Source: CAD feature listing. Evaluate the final solid. Frame: model axes, mm. A direction names the side the tool comes from. Round coordinates to 2 decimals unless told otherwise and drop trailing zeros. Loops run counter-clockwise (first coordinate to the right, second up) from the corner with the lowest first, then second, coordinate; pieces in that order, holes last. Notation, with made-up numbers: M 1,-28.75 L 32,-28.75 A18 cw 32,-19.75 Z; hole C 7,-37 d9. An arc over 180 degrees is marked long. Write each question's results on one line, items separated by ' | '. Start each with the question number.
1. Section B-B on x = 0. Output: boundary loops of the cut face in (y, z), and give its area (3 significant figures).
2. Set-up query: faces 1 (the flat face through (-1, 1, 3)), 2 (the flat face through (12.5, -5, -1)), 3 (the flat face through (-12.5, -5, -1)), 4 (the flat face through (12.5, 13, 1)). Return all of +Z, -Z, +X, -X, +Y, -Y with unobstructed straight access to the full face (end or side cutting, diameter ignored); none if empty.
3. Contact query for flat-ended pins moving along their axis: pin 1 Ø24 at (x, y) = (16, -10) entering from -Z; pin 2 Ø1 at (y, z) = (19, 1.5) entering from -X; pin 3 Ø2 at (y, z) = (29.5, 0.5) entering from -X; pin 4 Ø2.5 at (x, z) = (5.5, 1) entering from +Y. Output: stop coordinate, or through.
4. Section D-D on y = 12.5. Output: boundary loops of the cut face in (x, z), and give its area (3 significant figures).
5. Draft query along Y for faces 5 (the flat face through (0, 4, -1)), 6 (the flat face through (0, -5, -2)), 7 (the flat face through (0, 16.5, 1)), 8 (the flat face through (0, -14.5, -1)). Return one class per face: released by +Y, released by -Y, zero draft, split by the parting line, or undercut.
6. Section A-A on y = 0. Output: boundary loops of the cut face in (x, z).
7. Ray query, line 1 (X direction, y = 0, z = -0.45); line 2 (Y direction, x = -10.5, z = -0.2); line 3 (X direction, y = -12.5, z = 1.4). Return the intervals inside material, ascending.
8. Section C-C on z = -0.9. Output: boundary loops of the cut face in (x, y).
from build123d import *

# Parameters (mm, degrees)
ESQUISSE1_R                  = 40
ESQUISSE1_R_2                = 1.05
BOSS_EXTRU_1_DEPTH           = 3
ESQUISSE2_W                  = 25
ESQUISSE2_H                  = 7
ENL_V_MAT_EXTRU_4_DEPTH      = 14
BOSS_EXTRU_6_DEPTH           = 2
ENL_V_MAT_EXTRU_5_DEPTH      = 2
ESQUISSE2_9_W                = 12.5
ESQUISSE2_9_H                = 18.5
BOSS_EXTRU_7_DEPTH           = 2
ENL_V_MAT_EXTRU_6_DEPTH      = 57.648036153
ENL_V_MAT_EXTRU_6_DEPTH_BACK = 57.648036153
ESQUISSE7_R                  = 1.05


with BuildPart() as part:
    # Esquisse1 → Boss.-Extru.1 (new body)
    with BuildSketch(Plane.XY):
        Circle(ESQUISSE1_R)
        with Locations((-10.5, -12.5)):
            Circle(ESQUISSE1_R_2, mode=Mode.SUBTRACT)
        with Locations((10.5, -12.5)):
            Circle(ESQUISSE1_R_2, mode=Mode.SUBTRACT)
        with Locations((-10.5, 0)):
            Circle(ESQUISSE1_R_2, mode=Mode.SUBTRACT)
        with Locations((10.5, 0)):
            Circle(ESQUISSE1_R_2, mode=Mode.SUBTRACT)
    extrude(amount=BOSS_EXTRU_1_DEPTH)

    # Esquisse2 → Enl_v. mat.-Extru.4 (cut)
    with BuildSketch(Plane.XY):
        with Locations((0, 13)):
            Rectangle(ESQUISSE2_W, ESQUISSE2_H)
    extrude(amount=ENL_V_MAT_EXTRU_4_DEPTH, mode=Mode.SUBTRACT)

    # Esquisse2_7 → Boss.-Extru.6 (add)
    with BuildSketch(Plane.XY):
        Polygon((12.5, 4), (12.5, 9.5), (-12.5, 9.5), (-12.5, 4), (0, 4), align=None)
    extrude(amount=-BOSS_EXTRU_6_DEPTH)

    # Esquisse2_8 → Enl_v. mat.-Extru.5 (cut)
    with BuildSketch(Plane.XY):
        Polygon((12.5, 4), (12.5, 9.5), (-12.5, 9.5), (-12.5, 4), (0, 4), align=None)
    extrude(amount=-ENL_V_MAT_EXTRU_5_DEPTH, mode=Mode.SUBTRACT)

    # Esquisse2_9 → Boss.-Extru.7 (add)
    with BuildSketch(Plane.XY):
        with Locations((6.25, -5.25)):
            Rectangle(ESQUISSE2_9_W, ESQUISSE2_9_H)
        with Locations((-6.25, -5.25)):
            Rectangle(ESQUISSE2_9_W, ESQUISSE2_9_H)
    extrude(amount=-BOSS_EXTRU_7_DEPTH)

    # Esquisse7 → Enl_v. mat.-Extru.6 (cut, two sides: drawn at the far end of the back side and taken through both)
    with BuildSketch(Plane.XY.offset(-ENL_V_MAT_EXTRU_6_DEPTH_BACK)):
        with Locations((-10.5, 0)):
            Circle(ESQUISSE7_R)
        with Locations((-10.5, -12.5)):
            Circle(ESQUISSE7_R)
        with Locations((10.5, 0)):
            Circle(ESQUISSE7_R)
        with Locations((10.5, -12.5)):
            Circle(ESQUISSE7_R)
    extrude(amount=ENL_V_MAT_EXTRU_6_DEPTH + ENL_V_MAT_EXTRU_6_DEPTH_BACK, mode=Mode.SUBTRACT)


solid = part.part
Taken from the geometry:
1) outline: M -40,0 L -14.5,0 L -14.5,-2 L 4,-2 L 4,0 L 9.5,0 L 9.5,3 L -40,3 Z; M 16.5,0 L 40,0 L 40,3 L 16.5,3 Z | area: 256 mm^2
2) face 1: +Z, +X, -X, +Y, -Y | face 2: -Z, +X, +Y, -Y | face 3: -Z, -X, +Y, -Y | face 4: +Z, -Z
3) pin 1: z = -2 | pin 2: x = -35.46 | pin 3: x = -28.07 | pin 4: y = 39.77
4) outline: M -38,0 L -12.5,0 L -12.5,3 L -38,3 Z; M 12.5,0 L 38,0 L 38,3 L 12.5,3 Z | area: 153 mm^2
5) face 5: released by +Y | face 6: zero draft | face 7: undercut | face 8: released by -Y
6) outline: M -40,0 L -12.5,0 L -12.5,-2 L -11.55,-2 L -11.55,3 L -40,3 Z; M -9.45,-2 L 9.45,-2 L 9.45,3 L -9.45,3 Z; M 11.55,-2 L 12.5,-2 L 12.5,0 L 40,0 L 40,3 L 11.55,3 Z
7) line 1: -12.5 to -11.55, -9.45 to 9.45, 11.55 to 12.5 | line 2: -14.5 to -13.55, -11.45 to -1.05, 1.05 to 4 | line 3: -38 to -11.55, -9.45 to 9.45, 11.55 to 38
8) outline: M -12.5,-14.5 L 12.5,-14.5 L 12.5,4 L -12.5,4 Z; hole C -10.5,-12.5 d2.1; hole C -10.5,0 d2.1; hole C 10.5,-12.5 d2.1; hole C 10.5,0 d2.1
